For this review, use the dimensioned drawing (mm, ordinates from the lowest corner) and the shaded views. Coordinates: 2 decimals unless noted, no trailing zeros. Loops run counter-clockwise (first coordinate to the right, second up) from the corner with the lowest first, then second, coordinate; pieces in that order, holes last. Notation, with made-up numbers: (46, 12) - (93, 12) arc R30 ccw to (93, 43) - close; hole circle Ø8 at (4, 82). An arc over 180 degrees is marked (long way). Answer in a Markdown table with one row per item. Add a question column.
(1) For P1, Ø0.6, axis at x = 5, y = 1.5, coming from the -Z side; P2, Ø5, axis at x = 18, z = 16.5, coming from the -Y side; P3, Ø6, axis at x = 27.5, z = 8.5, coming from the +Y side; P4, Ø0.6, axis at x = 2, y = 1.5, coming from the +Z side, all flat-tipped, find the tip position at first contact; note any pin that passes through.
(2) For line 1 along X through (y, z) = (0.15, 13); line 2 along Z through (x, y) = (17, 0.3); line 3 along Z through (x, y) = (28, 1.6), list the stretches that pass through material, from the lowest coordinate up.
(3) We need section D-D on x = 20.5. Write out the cut boundary in (y, z).
(4) We need section B-B on y = 1.35. Write out the cut boundary in (x, z) (1 decimal).
(5) We need section A-A on z = 19.5. Write out the cut boundary in (x, y) (1 decimal).
(6) We need section C-C on x = 31. Write out the cut boundary in (y, z).
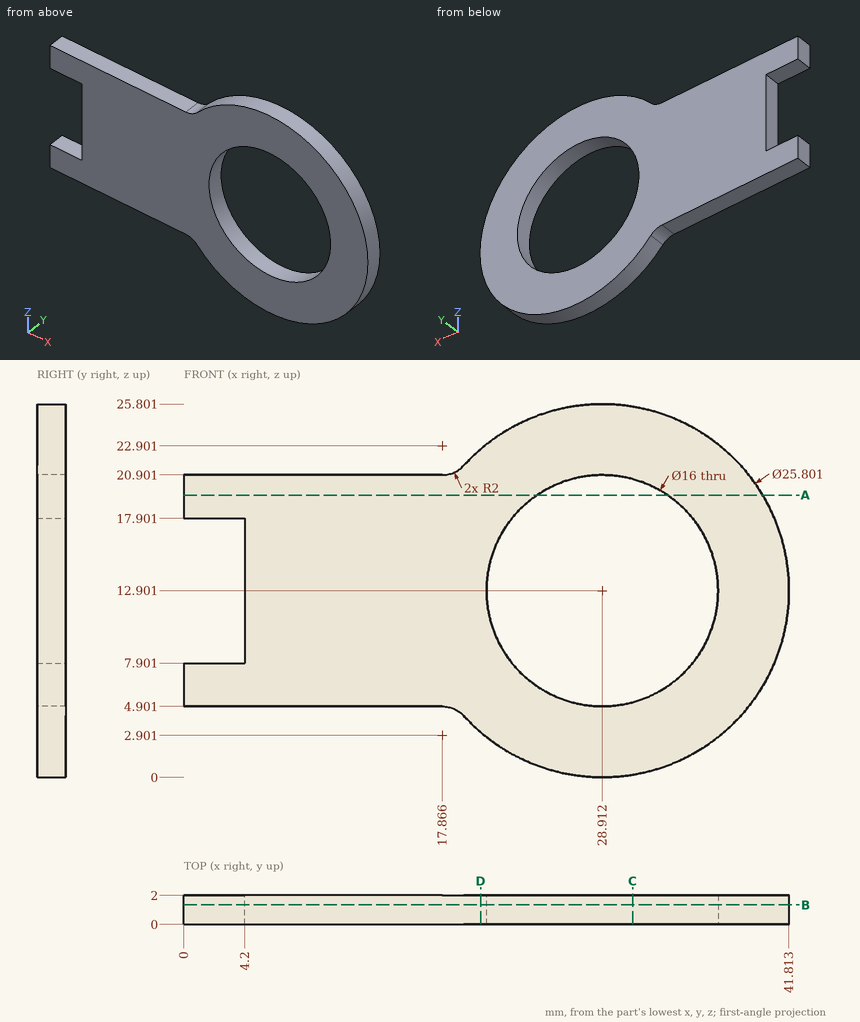
Outcome:
| question | item | result |
|---|---|---|
| 1 | P1 | z = 4.9 |
| 1 | P2 | y = 0 |
| 1 | P3 | through |
| 1 | P4 | z = 20.9 |
| 2 | line 1 | 4.2 to 20.91, 36.91 to 41.81 |
| 2 | line 2 | 4.9 to 20.9 |
| 2 | line 3 | 0.03 to 4.95, 20.85 to 25.77 |
| 3 | outline | (0, 3.12) - (2, 3.12) - (2, 22.68) - (0, 22.68) - close |
| 4 | outline | (0, 4.9) - (17.9, 4.9) arc R2 cw to (19.3, 4.2) arc R12.9 ccw (long way) to (19.3, 21.6) arc R2 cw to (17.9, 20.9) - (0, 20.9) - (0, 17.9) - (4.2, 17.9) - (4.2, 7.9) - (0, 7.9) - close; hole circle Ø16 at (28.9, 12.9) |
| 5 | outline | (0, 0) - (24.4, 0) - (24.4, 2) - (0, 2) - close; (33.4, 0) - (40, 0) - (40, 2) - (33.4, 2) - close |
| 6 | outline | (0, 0.17) - (2, 0.17) - (2, 5.18) - (0, 5.18) - close; (0, 20.62) - (2, 20.62) - (2, 25.63) - (0, 25.63) - close |
